Here's how the part is built. I have some questions about the finished solid (model axes, mm). A direction names the side the tool comes from. Round coordinates to 2 decimals unless told otherwise and drop trailing zeros. Write each loop counter-clockwise with the first axis right and the second up, starting at its lowest first coordinate (ties: lowest second). Pieces come first, ordered by that corner, then holes. Notation, with made-up numbers: M -33.5,-34 L -10.5,-34 A8 ccw -10.5,-27 Z; hole C -31,47.5 d3. An arc over 180 degrees is marked long. Use a Markdown table: item, result. Add a question column.
```python
from build123d import *

# Parameters (mm, degrees)
BOSS_EXTRUDE1_DEPTH     = 36.5
CUT_EXTRUDE1_DEPTH      = 53.82281704
CUT_EXTRUDE1_DEPTH_BACK = 3.2
CUT_EXTRUDE1_START      = 36.5
SKETCH2_W               = 57.250046972
SKETCH2_H               = 6


with BuildPart() as part:
    # Sketch1 → Boss-Extrude1 (new, symmetric)
    with BuildSketch(Plane(origin=(0, 0, 0), x_dir=(0, 0, -1), z_dir=(1, 0, 0))):
        with BuildLine():
            Line((-27, 0), (-23, 0))
            ThreePointArc((-23, 0), (0, -23), (23, 0))
            Line((23, 0), (27, 0))
            ThreePointArc((27, 0), (0, -27), (-27, 0))
        make_face()
    extrude(amount=BOSS_EXTRUDE1_DEPTH, both=True)

    # Sketch2 → Cut-Extrude1 (cut, two sides: drawn at the far end of the back side and taken through both)
    with BuildSketch(Plane(origin=(0, 0, 0), x_dir=(0, 0, -1), z_dir=(1, 0, 0)).offset(CUT_EXTRUDE1_START - CUT_EXTRUDE1_DEPTH_BACK)):
        with Locations((-0.586463896, -9)):
            Rectangle(SKETCH2_W, SKETCH2_H)
    extrude(amount=CUT_EXTRUDE1_DEPTH + CUT_EXTRUDE1_DEPTH_BACK, mode=Mode.SUBTRACT)


solid = part.part
```
Item 1: If we mould it in two halves opening along Y, with no side actions, what happens to faces 1 (the face through (0.511, -22.994, 0.506)), 2 (the face through (36.5, -24, 0)), 3 (the face through (35, -6, 24))? For each: +Y half, -Y half, draft (parallel to the pull), parting line (faces both ways), or undercut.
Item 2: Imagine slicing it at A-A on y = -14.5. List the corners of the cut face in (x, z) for me, plus the area to 3 significant figures.
Item 3: Imagine slicing it at C-C on x = 32.5. List the corners of the cut face in (y, z) for me, plus the area to 3 significant figures.
Item 4: Imagine slicing it at B-B on z = 0. List the corners of the cut face in (x, y) for me, plus the area to 3 significant figures.
Item 5: Imagine slicing it at D-D on y = -8.25. List the corners of the cut face in (x, z) for me.
Item 6: I need wall thicknesses on probe 1 along Z at (x, y) = (-30, -15.25); probe 2 along Z at (x, y) = (-3.5, -18.75); probe 3 along Y at (x, z) = (14, 7). Which ranges of each line are inside material? Lowest first, please. Write a range as from..to.
Item 7: For pin 1 Ø12 at (y, z) = (-9, -8.5) entering from -X; pin 2 Ø1.6 at (x, z) = (34.5, 24) entering from -Y; pin 3 Ø1.8 at (y, z) = (-8, -23) entering from +X; pin 4 Ø2.5 at (x, z) = (35, -23.5) entering from -Y (3 decimals), each with a flat end and sliding along its axis, tell me the tip position at first contact or that it passes through.
Item 8: On a 3-axis mill with a long thin cutter (end or side, diameter ignored), from which of +Z, -Z, +X, -X, +Y, -Y can I reach the whole of each face in a straight line? I mean faces 4 (the face through (35, -12, 22)), 5 (the face through (36.5, -3, 25)). Say none if no direction works.
The answers:
| question | item | result |
|---|---|---|
| 1 | face 1 | +Y half |
| 1 | face 2 | draft |
| 1 | face 3 | undercut |
| 2 | outline | M -36.5,-22.78 L 36.5,-22.78 L 36.5,-17.85 L -36.5,-17.85 Z; M -36.5,17.85 L 36.5,17.85 L 36.5,22.78 L -36.5,22.78 Z |
| 2 | area | 719 mm² |
| 3 | outline | M 0,-27 L 0,-23 A23 cw 0,23 L 0,27 A27 ccw Z |
| 3 | area | 314 mm² |
| 4 | outline | M -36.5,-27 L 36.5,-27 L 36.5,-23 L -36.5,-23 Z |
| 4 | area | 292 mm² |
| 5 | outline | M -36.5,-25.71 L 33.3,-25.71 L 33.3,-21.47 L -36.5,-21.47 Z; M -36.5,21.47 L 33.3,21.47 L 33.3,25.71 L -36.5,25.71 Z |
| 6 | probe 1 | -22.28..-17.22, 17.22..22.28 |
| 6 | probe 2 | -19.43..-13.32, 13.32..19.43 |
| 6 | probe 3 | -26.08..-21.91 |
| 7 | pin 1 | through |
| 7 | pin 2 | y = -13.81 |
| 7 | pin 3 | x = 33.3 |
| 7 | pin 4 | y = -15.295 |
| 8 | face 4 | +Z, -Z, +X |
| 8 | face 5 | +Z, -Z, +X, +Y, -Y |
